```python
from build123d import *

# Parameters (mm, degrees)
SKETCH1_W               = 3.3
SKETCH1_H               = 7.4
SKETCH1_W_2             = 18
SKETCH1_H_2             = 1.6
BOSS_EXTRUDE1_DEPTH     = 2.6
SKETCH3_W               = 18
SKETCH3_H               = 22.9
BOSS_EXTRUDE2_DEPTH     = 1.6
CUT_EXTRUDE1_DEPTH      = 27.511924597
CUT_EXTRUDE1_DEPTH_BACK = 27.511924597
FILLET1_R               = 2
FILLET2_R               = 1
BOSS_EXTRUDE3_DEPTH     = 5
CUT_EXTRUDE2_DEPTH      = 10


with BuildPart() as part:
    # Sketch1 → Boss-Extrude1 (new body)
    with BuildSketch(Plane.XY):
        with Locations((0.442709082, -7.556371191)):
            Rectangle(SKETCH1_W, SKETCH1_H)
        with Locations((7.792709082, -7.556371191)):
            Rectangle(SKETCH1_W, SKETCH1_H)
        with Locations((0.442709082, 3.093628809)):
            Rectangle(SKETCH1_W_2, SKETCH1_H_2)
        with Locations((0.442709082, -18.206371191)):
            Rectangle(SKETCH1_W_2, SKETCH1_H_2)
        with Locations((0.442709082, -7.556371191)):
            Rectangle(SKETCH1_W_2, SKETCH1_H)
    extrude(amount=BOSS_EXTRUDE1_DEPTH)

    # Sketch3 → Boss-Extrude2 (add)
    with BuildSketch(Plane.XY.offset(2.6)):
        with Locations((0.442709082, -7.556371191)):
            Rectangle(SKETCH3_W, SKETCH3_H)
    extrude(amount=BOSS_EXTRUDE2_DEPTH)

    # Sketch4 → Cut-Extrude1 (cut, two sides: drawn at the far end of the back side and taken through both)
    with BuildSketch(Plane.ZY.offset(8.557290918).offset(-CUT_EXTRUDE1_DEPTH_BACK)):
        Polygon((1.342435563, -8.644254243), (0.613371363, -8.644254243), (0.977903463, -9.008786343), align=None)
        Polygon((2.430318615, -7.556371191), (1.342435563, -6.468488139), (1.342435563, -8.644254243), align=None)
        Polygon((0.977903463, -6.103956039), (0.613371363, -6.468488139), (1.342435563, -6.468488139), align=None)
        Polygon((0.613371363, -6.468488139), (0, -7.081859502), (0, -8.03088288), (0.613371363, -8.644254243), (1.342435563, -8.644254243), (1.342435563, -6.468488139), align=None)
        Polygon((0, -6.468488139), (0, -7.081859502), (0.613371363, -6.468488139), align=None)
        Polygon((0.613371363, -8.644254243), (0, -8.03088288), (0, -8.644254243), align=None)
    extrude(amount=CUT_EXTRUDE1_DEPTH + CUT_EXTRUDE1_DEPTH_BACK, mode=Mode.SUBTRACT)

    # Fillet1
    fillet1_edges = [part.edges().sort_by_distance(p)[0] for p in [
        (9.442709082, 3.893628809, 2.1),
        (9.442709082, -19.006371191, 2.1),
    ]]
    fillet(fillet1_edges, radius=FILLET1_R)

    # Fillet2
    fillet2_edges = [part.edges().sort_by_distance(p)[0] for p in [
        (9.442709082, -7.556371191, 4.2),
        (8.856922645, -18.420584754, 4.2),
        (8.856922645, 3.307842371, 4.2),
        (-8.557290918, -7.556371191, 4.2),
        (-0.557290918, -19.006371191, 4.2),
        (-0.557290918, 3.893628809, 4.2),
    ]]
    fillet(fillet2_edges, radius=FILLET2_R)

    # Sketch6 → Boss-Extrude3 (add)
    with BuildSketch(Plane(origin=(9.442709082, 0, 0), x_dir=(0, 0, -1), z_dir=(1, 0, 0))):
        Polygon((-2.6, -3.856371191), (-2.6, -11.256371191), (0, -11.256371191), (0, -8.644254243), (-0.613371363, -8.644254243), (-0.977903463, -9.008786343), (-2.430318615, -7.556371191), (-0.977903463, -6.103956039), (-0.613371363, -6.468488139), (0, -6.468488139), (0, -3.856371191), align=None)
    extrude(amount=BOSS_EXTRUDE3_DEPTH)

    # Sketch5 → Cut-Extrude2 (cut)
    with BuildSketch(Plane.XZ.offset(11.256371191)):
        Polygon((-5.257290918, 2.6), (-1.207290918, 2.6), (1.809394507, -0.416685424), (-2.240605493, -0.416685424), align=None)
        Polygon((2.092709082, 2.6), (6.142709082, 2.6), (10.446710416, -1.704001333), (6.396710416, -1.704001333), align=None)
        Polygon((-8.557290918, 2.6), (-13.200539382, 2.6), (-10.121786084, -0.478753297), (-5.47853762, -0.478753297), align=None)
        Polygon((9.442709082, 2.6), (15.456496685, 2.6), (19.467588869, -1.411092184), (13.453801266, -1.411092184), align=None)
    extrude(amount=-CUT_EXTRUDE2_DEPTH, mode=Mode.SUBTRACT)


solid = part.part
```
CAD build for the part. Positions are in the model's coordinates, mm. A direction names the side the tool comes from. Coordinates: 2 decimals unless noted, no trailing zeros. Write each loop counter-clockwise with the first axis right and the second up, starting at its lowest first coordinate (ties: lowest second). Pieces come first, ordered by that corner, then holes.
(1) Drill centre lines: probe 1 along Y at (x, z) = (6, 0.4); probe 2 along Y at (x, z) = (-5.5, 1.45); probe 3 along X at (y, z) = (-7, 2.25). Where is each one in solid material? Low to high.
(2) Two-plate mould, pull along Y, no slides. Class faces 5 (the face through (2.83, -8.43, 1.86)), 6 (the face through (-8.557, -8, 3)), 7 (the face through (-0.669, 3.593, 3.915)): +Y half, -Y half, draft (parallel to the pull), parting line (faces both ways), or undercut.
(3) Cut at A-A, the plane z = 0.3. Count the separate pieces of the cut face and the enclosed holes in it, and give its area (3 significant figures).
(4) Cut at B-B, the plane x = -4.5. List the corners of the cut face in (y, z).
(5) 3-axis set-ups, long thin cutter, end or side, ignore diameter. For faces 1 (the face through (-7.82, -8.43, 1.86)), 2 (the face through (10, -5, 0)), 3 (the face through (0, -17.406, 1)), 4 (the face through (-6.045, -8.293, 1.694)): which of +Z, -Z, +X, -X, +Y, -Y reach the whole face in a straight line?
(6) Flat gauge pins, fed straight in: pin 1 (2 mm diameter, centred on x = 9, z = 2, fed in from +Y); pin 2 (1.3 mm diameter, centred on x = 9.5, z = 1, fed in from -Y); pin 3 (0.5 mm diameter, centred on x = 11, z = 0, fed in from -Y); pin 4 (1.5 mm diameter, centred on y = -14, z = 3.5, fed in from -X). Where does each tip first touch, or does it go through?
(7) Cut at C-C, the plane y = -1.25. List the corners of the cut face in (x, z), and give its area (3 significant figures).
(8) Cut at D-D, the plane x = 5.75. List the corners of the cut face in (y, z).
Geometry says:
1. probe 1: y = -19.01 to -17.41, 2.29 to 3.89
1. probe 2: y = -19.01 to -17.41, -11.26 to -8.54, -6.58 to -3.86, 2.29 to 3.89
1. probe 3: x = -8.21 to -4.91, -0.86 to 2.44, 6.49 to 9.79
2. face 5: undercut
2. face 6: draft
2. face 7: +Y half
3. separate pieces: 8
3. enclosed holes: 0
3. area: 108 mm2
4. outline: (-19.01, 0) - (-17.41, 0) - (-17.41, 2.6) - (2.29, 2.6) - (2.29, 0) - (3.89, 0) - (3.89, 3.2) arc R1 ccw to (2.89, 4.2) - (-18.01, 4.2) arc R1 ccw to (-19.01, 3.2) - close; (-11.26, 0) - (-8.64, 0) - (-8.64, 0.61) - (-9.01, 0.98) - (-8.14, 1.84) - (-11.26, 1.84) - close; (-6.97, 1.84) - (-6.1, 0.98) - (-6.47, 0.61) - (-6.47, 0) - (-3.86, 0) - (-3.86, 1.84) - close
5. face 1: -Z, -X
5. face 2: -Z, +X, -X, +Y, -Y
5. face 3: -Z, +X, -X
5. face 4: +X, -X
6. pin 1: stops at y = 3.81
6. pin 2: stops at y = -18.43
6. pin 3: stops at y = -11.26
6. pin 4: stops at x = -8.56
7. outline: (-8.56, 2.6) - (9.44, 2.6) - (9.44, 3.2) arc R1 ccw to (8.44, 4.2) - (-7.56, 4.2) arc R1 ccw to (-8.56, 3.2) - close
7. area: 28.4 mm2
8. outline: (-19.01, 0) - (-17.41, 0) - (-17.41, 2.6) - (2.29, 2.6) - (2.29, 0) - (3.89, 0) - (3.89, 3.2) arc R1 ccw to (2.89, 4.2) - (-18.01, 4.2) arc R1 ccw to (-19.01, 3.2) - close
